```python
from build123d import *

# Parameters (mm, degrees)
F0_W     = 100
F0_H     = 100
F1_DEPTH = 10
F3_DEPTH = 25
F5_DEPTH = 25


with BuildPart() as f1:
    # F0 (on Top) → F1 (new body)
    with BuildSketch(Plane.XY):
        Rectangle(F0_W, F0_H)
    extrude(amount=F1_DEPTH)

    # F2 (on Top) → F3 (join)
    with BuildSketch(Plane.XY):
        Polygon((34.999999, -10), (-10, -10), (-10, 34.999999), (-15.000001, 34.999999), (-15.000001, -15.000001), (34.999999, -15.000001), align=None)
    extrude(amount=-F3_DEPTH)

    # F4 (on Top) → F5 (cut)
    with BuildSketch(Plane.XY):
        with BuildLine():
            ThreePointArc((-7.5, 0), (0, -7.5), (7.5, 0))
            ThreePointArc((7.5, 0), (0, 7.5), (-7.5, 0))
        make_face()
        with BuildLine():
            ThreePointArc((-7.5, 0), (0, 7.5), (7.5, 0))
            Line((7.5, 0), (7.5, 35))
            ThreePointArc((7.5, 35), (0, 27.5), (-7.5, 35))
            Line((-7.5, 35), (-7.5, 0))
        make_face()
        with BuildLine():
            ThreePointArc((-7.5, 35), (0, 27.5), (7.5, 35))
            ThreePointArc((7.5, 35), (0, 42.5), (-7.5, 35))
        make_face()
    extrude(amount=F5_DEPTH, mode=Mode.SUBTRACT)


solid = f1.part
```
Design review of the part built by this model. Coordinates are the model's own, in mm. A direction names the side the tool comes from. Coordinates: 2 decimals unless noted, no trailing zeros. Order: outer loops, then holes, each group sorted by start corner. A loop starts at its lowest first (then second) coordinate and runs counter-clockwise, first axis right, second up.
1) Take a section at A-A, the plane y = 12.5. Give the boundary of the cut face in (x, z).
2) Clearance check with flat-ended pins moving along their axes: pin 1 (4 mm diameter, centred on x = -12, z = -10, fed in from +Y); pin 2 (1 mm diameter, centred on y = 26, z = -9, fed in from +X); pin 3 (6 mm diameter, centred on x = 36.5, z = -21, fed in from +Y). State where each tip first meets the part, or that it passes through.
3) Take a section at C-C, the plane z = 5.5. Give the boundary of the cut face in (x, y), and give its area (3 significant figures).
4) Mouldability with a two-part tool opening along X and no side actions: class faces 5 (the flat face through (-1.2, -10.3, -25)), 6 (the flat face through (35, -13, -12)), 7 (the flat face through (7.5, 17, 5)) as +X half, -X half, draft (parallel to the pull), parting line (faces both ways), or undercut.
5) For faces 1 (the flat face through (-12, 35, -12)), 2 (the flat face through (-15, 10, -12)), 3 (the flat face through (-10, 12, -12)), 4 (the cylindrical face through (0.16, 42.5, 4.93)), list the 3-axis set-ups (+Z, -Z, +X, -X, +Y, -Y) from which the entire face can be reached by the end or side of a thin tool; tool diameter is ignored.
6) Take a section at D-D, the plane x = 23. Give the boundary of the cut face in (y, z).
7) Take a section at B-B, the plane x = 0. Give the boundary of the cut face in (y, z), and give its area (3 significant figures).
8) Wall thickness on line 1 along X through (y, z) = (26.5, 2); line 2 along Z through (x, y) = (-17.5, 21); line 3 along X through (y, z) = (9.5, -18): over which ranges is each line inside the solid? List them lowest first.
Returned:
1. outline: (-50, 0) - (-15, 0) - (-15, -25) - (-10, -25) - (-10, 0) - (-7.5, 0) - (-7.5, 10) - (-50, 10) - close; (7.5, 0) - (50, 0) - (50, 10) - (7.5, 10) - close
2. pin 1: stops at y = 35
2. pin 2: stops at x = -10
2. pin 3: stops at y = -10
3. outline: (-50, -50) - (50, -50) - (50, 50) - (-50, 50) - close; hole (-7.5, 0) arc R7.5 ccw to (7.5, 0) - (7.5, 35) arc R7.5 ccw to (-7.5, 35) - close
3. area: 9,300 mm2
4. face 5: draft
4. face 6: +X half
4. face 7: undercut
5. face 1: -Z, +X, -X, +Y
5. face 2: -Z, -X, +Y, -Y
5. face 3: -Z, +X, +Y
5. face 4: +Z, -Z
6. outline: (-50, 0) - (-15, 0) - (-15, -25) - (-10, -25) - (-10, 0) - (50, 0) - (50, 10) - (-50, 10) - close
7. outline: (-50, 0) - (-15, 0) - (-15, -25) - (-10, -25) - (-10, 0) - (-7.5, 0) - (-7.5, 10) - (-50, 10) - close; (42.5, 0) - (50, 0) - (50, 10) - (42.5, 10) - close
7. area: 625 mm2
8. line 1: x = -50 to -7.5, 7.5 to 50
8. line 2: z = 0 to 10
8. line 3: x = -15 to -10
